Answer from the drawing. Dimensions are ordinates in mm from the lowest x, y and z of the part. A direction names the side the tool comes from. Round coordinates to 2 decimals unless told otherwise and drop trailing zeros. Order: outer loops, then holes, each group sorted by start corner. A loop starts at its lowest first (then second) coordinate and runs counter-clockwise, first axis right, second up. Notation, with made-up numbers: M -18,73 L 21,73 A21 ccw 21,89 Z; hole C 22.5,-10.75 d3. An arc over 180 degrees is marked long. Write item = value, one per line. Start each with the question number.
(1) A cutting plane is placed at D-D, the plane x = 1.5. Determine the outline of the cut face in (y, z), and give its area (3 significant figures).
(2) Straight lines are drawn through the part: probe 1 along Z at (x, y) = (5, 5.75); probe 2 along Z at (x, y) = (17.5, 1.15); probe 3 along Y at (x, z) = (20, 58). For each, find the intervals that lie inside material, in ascending order. Write a range as from..to.
(3) Which of the six approach directions +Z, -Z, +X, -X, +Y, -Y give full straight-line access (tool end or side, diameter ignored) to the marked faces 4 and 5?
(4) A cutting plane is placed at C-C, the plane y = 3.5. Determine the outline of the cut face in (x, z).
(5) For a pull along Z with two mould halves and no side action, classify the marked faces 1, 2 and 3 as released by +Z, released by -Z, zero draft, split by the parting line, or undercut.
(6) Each of these flat-tipped pins is pushed along its axis until it touches: pin 1 (10 mm diameter, centred on x = 13, z = 43, fed in from +Y); pin 2 (0.7 mm diameter, centred on y = 1, z = 45.5, fed in from -X). Where does it stop, or does it pass through?
(7) A cutting plane is placed at A-A, the plane z = 10. Determine the outline of the cut face in (x, y).
(8) A cutting plane is placed at B-B, the plane x = 19. Determine the outline of the cut face in (y, z).
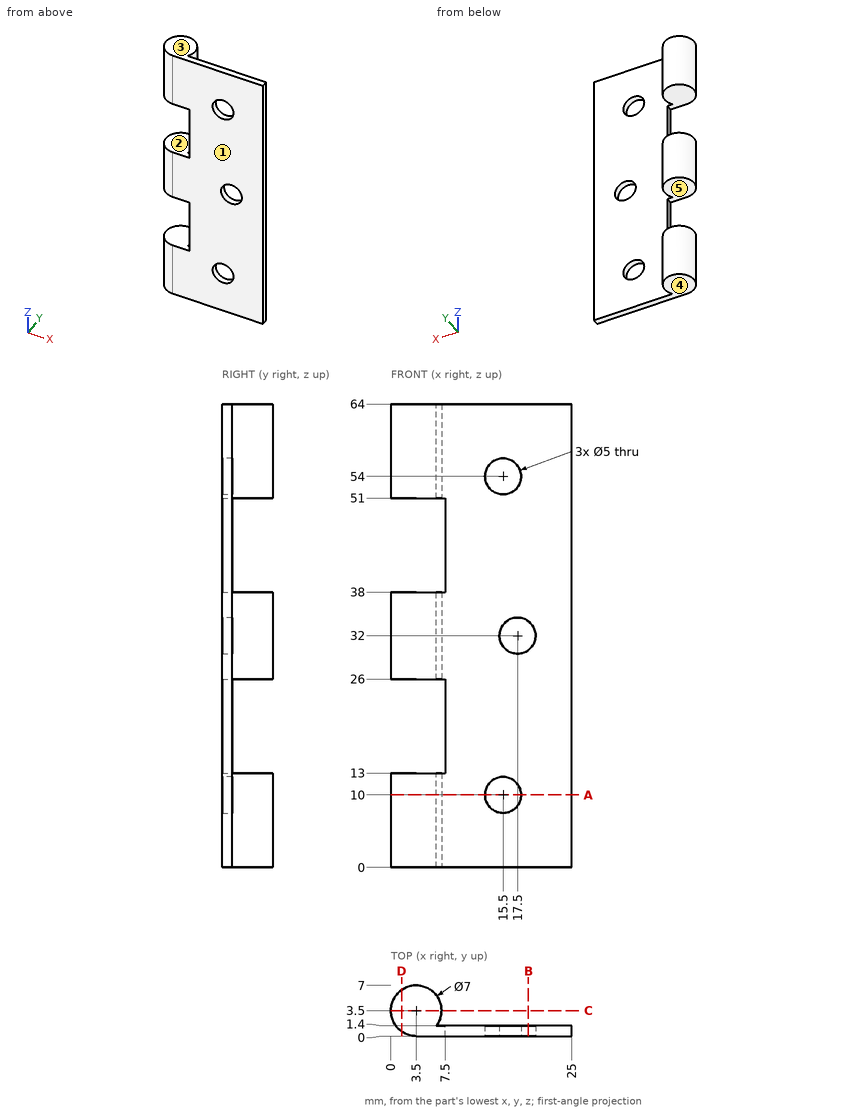
Reported:
q1.outline = M 0.63,0 L 6.37,0 L 6.37,13 L 0.63,13 Z; M 0.63,26 L 6.37,26 L 6.37,38 L 0.63,38 Z; M 0.63,51 L 6.37,51 L 6.37,64 L 0.63,64 Z
q1.area = 218 mm²
q2.probe_1 = 0..13, 26..38, 51..64
q2.probe_2 = 0..8.5, 11.5..29.5, 34.5..52.5, 55.5..64
q2.probe_3 = 0..1.4
q3.face_4 = -Z, +X, -X, +Y, -Y
q3.face_5 = -X, +Y, -Y
q4.outline = M 0,0 L 7,0 L 7,13 L 0,13 Z; M 0,26 L 7,26 L 7,38 L 0,38 Z; M 0,51 L 7,51 L 7,64 L 0,64 Z
q5.face_1 = zero draft
q5.face_2 = undercut
q5.face_3 = released by +Z
q6.pin_1 = 1.4
q6.pin_2 = 7.5
q7.outline = M 3.5,0 L 13,0 L 13,1.4 L 6.3,1.4 A3.5 ccw long Z; M 18,0 L 25,0 L 25,1.4 L 18,1.4 Z
q8.outline = M 0,0 L 1.4,0 L 1.4,30 L 0,30 Z; M 0,34 L 1.4,34 L 1.4,64 L 0,64 Z
